The drawing under review shows one solid part. Ordinate dimensions are in mm from its lowest x, y, z. Give positions to 0.01 mm unless a question says otherwise; leave off trailing zeros. Write each loop counter-clockwise with the first axis right and the second up, starting at its lowest first coordinate (ties: lowest second). Pieces come first, ordered by that corner, then holes. Notation, with made-up numbers: M -14,37.25 L 12,37.25 A22 cw 12,62.25 Z; hole C 61.25,50.5 d3. An arc over 180 degrees is marked long. One line per item, written item: value. Start each with the question number.
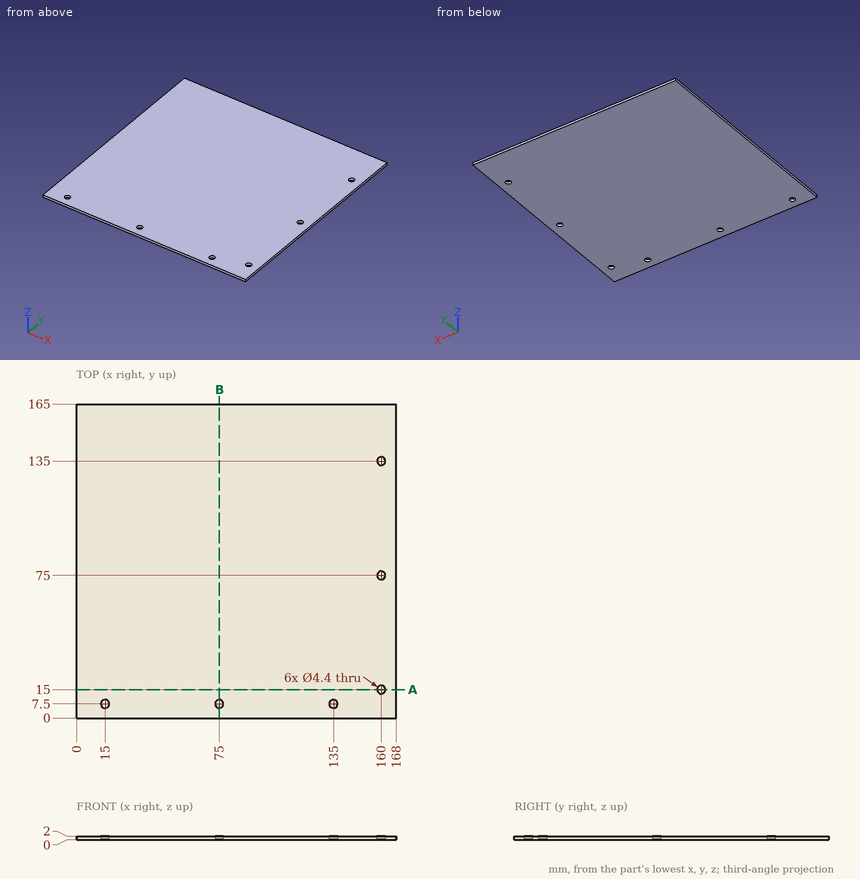
Q1. Wall thickness on line 1 (Y direction, x = 160, z = 0.8); line 2 (Y direction, x = 15, z = 0.65); line 3 (Y direction, x = 159.5, z = 1.65): over which ranges is each line inside the solid? List them lowest first. Write a range as from..to.
Q2. Take a section at B-B, the plane x = 75. Give the boundary of the cut face in (y, z), then the cut area to 3 significant figures.
Q3. Take a section at A-A, the plane y = 15. Give the boundary of the cut face in (x, z), then the cut area to 3 significant figures.
Q4. For P1, Ø2.5, axis at x = 160, y = 75, coming from the +Z side, flat-tipped, find the tip position at first contact; note if it passes through.
Results list:
1. line 1: y = 0..12.8, 17.2..72.8, 77.2..132.8, 137.2..165
1. line 2: y = 0..5.3, 9.7..165
1. line 3: y = 0..12.86, 17.14..72.86, 77.14..132.86, 137.14..165
2. outline: M 0,0 L 5.3,0 L 5.3,2 L 0,2 Z; M 9.7,0 L 165,0 L 165,2 L 9.7,2 Z
2. area: 321 mm^2
3. outline: M 0,0 L 157.8,0 L 157.8,2 L 0,2 Z; M 162.2,0 L 168,0 L 168,2 L 162.2,2 Z
3. area: 327 mm^2
4. P1: passes through
